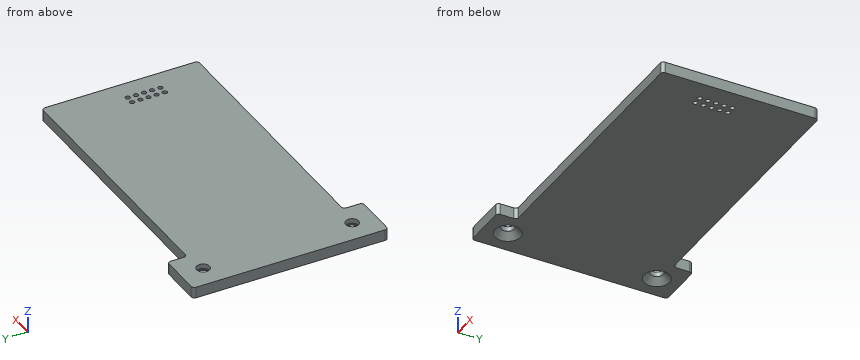
Autodesk Inventor part; units mm, degrees
ref_plane "YZ Plane" through (0, 0, 0) normal (1, 0, 0) x (0, 1, 0)
ref_plane "XZ Plane" through (0, 0, 0) normal (0, 1, 0) x (-1, 0, 0)
ref_plane "XY Plane" through (0, 0, 0) normal (0, 0, 1) x (1, 0, 0)
sketch "Boceto1" plane through (0, 0, 0) normal (0, 0, 1) x (1, 0, 0)
  line L0 (-26, 17) -> (26, 17)
  line L1 (26, 17) -> (26, -17)
  line L2 (26, -17) -> (-26, -17)
  line L3 (-26, -17) -> (-26, 17)
  line L4 (-26, 17) -> (26, -17) construction
  line L5 (26, 17) -> (-26, -17) construction
  point P0 (0, 0)
  dimension "d0" = 52
  dimension "d1" = 34
extrude "Extrusión1" add sketch "Boceto1" against normal blind 1.742
fillet "Empalme1" radius 0.5 4 edges at (26, 17, -0.871) (-26, 17, -0.871) (-26, -17, -0.871) (26, -17, -0.871)
sketch "Boceto2" plane through (0, 0, -1.742) normal (0, 0, -1) x (-1, 0, 0)
  line L0 (-25.5, 17) -> (25.5, 17)
  line L1 (25.5, -17) -> (-25.5, -17)
  line L2 (25.5, 17) -> (-25.5, 17)
  line L3 (15.5, 17) -> (-26, 17)
  line L4 (-26, 17) -> (-26, 12.2)
  line L5 (-26, 12.2) -> (15.5, 12.2)
  line L6 (15.5, 12.2) -> (15.5, 17)
  line L7 (-26, -16.5) -> (-26, 16.5)
  line L8 (-25.5, -17) -> (25.5, -17)
  line L9 (-26, 16.5) -> (-26, -16.5)
  line L10 (15.5, -17) -> (-26, -17)
  line L11 (-26, -17) -> (-26, -12.2)
  line L12 (-26, -12.2) -> (15.5, -12.2)
  line L13 (15.5, -12.2) -> (15.5, -17)
  point P0 (0, 0)
  dimension "d5" = 4.8
  dimension "d6" = 41.5
  dimension "d7" = 4.8
  dimension "d8" = 41.5
extrude "Extrusión2" cut sketch "Boceto2" against normal through all
sketch "Boceto4" plane through (0, 0, 0) normal (0, 0, 1) x (1, 0, 0)
  line L0 (-26, -16.5) -> (-26, 16.5) construction
  line L1 (-26, 17) -> (-22.8, 17)
  line L2 (-22.8, 17) -> (-22.8, -17)
  line L3 (-22.8, -17) -> (-26, -17)
  line L4 (-26, -17) -> (-26, 17)
  line L5 (-15.5, -17) -> (-25.5, -17)
  line L6 (-25.5, 17) -> (-15.5, 17)
  point P0 (0, 0)
  dimension "d17" = 3.2
extrude "Extrusión4" cut sketch "Boceto4" against normal up to surface (1.742 mm away)
sketch "Boceto7" plane through (0, 0, -1.742) normal (0, 0, -1) x (-1, 0, 0)
  line L0 (22.8, -17) -> (22.8, 17)
  line L1 (22.8, 17) -> (15.5, 17)
  line L2 (15.5, -17) -> (22.8, -17)
  point P0 (0, 0)
  point P1 (19.1, 11.638)
  point P2 (19.1, -11.638)
  dimension "d30" = 3.7
  dimension "d31" = 5.362
  dimension "d32" = 5.362
hole "Agujero2" at (-19.1, 11.638, -1.742) at (-19.1, -11.638, -1.742) direction (0, 0, 1) diameter 2 end through all countersink diameter 4 countersink angle 90
fillet "Empalme2" radius 0.5 8 edges at (-15.5, 17, -0.871) (-22.8, 17, -0.871) (-15.5, 12.2, -0.871) (26, 12.2, -0.871) (26, -12.2, -0.871) (-15.5, -12.2, -0.871) (-15.5, -17, -0.871) (-22.8, -17, -0.871)
sketch "Boceto8" plane through (0, 0, -1.742) normal (0, 0, -1) x (-1, 0, 0)
  line L0 (-26, 11.7) -> (-26, -11.7) construction
  line L1 (-25.5, -12.2) -> (15, -12.2) construction
  circle A0 centre (-22.735, 0.54) radius 0.37
  circle A1 centre (-21.465, 0.54) radius 0.37
  circle A2 centre (-22.735, -0.73) radius 0.37
  circle A3 centre (-21.465, -0.73) radius 0.37
  circle A4 centre (-22.735, -2) radius 0.37
  circle A5 centre (-21.465, -2) radius 0.37
  circle A6 centre (-22.735, -3.27) radius 0.37
  circle A7 centre (-21.465, -3.27) radius 0.37
  circle A8 centre (-22.735, -4.54) radius 0.37
  circle A9 centre (-21.465, -4.54) radius 0.37
  point P0 (0, 0)
  dimension "d49" = 3.265
  dimension "d50" = 1.27
  dimension "d51" = 1.27
  dimension "d52" = 1.27
  dimension "d53" = 1.27
  dimension "d54" = 12.74
  dimension "d55" = 0.74
  dimension "d56" = 0.74
  dimension "d57" = 0.74
  dimension "d58" = 0.74
  dimension "d59" = 0.74
  dimension "d60" = 0.74
  dimension "d61" = 0.74
  dimension "d62" = 0.74
  dimension "d63" = 1.27
  dimension "d64" = 0.74
  dimension "d65" = 0.74
extrude "Extrusión5" cut sketch "Boceto8" against normal up to surface (1.742 mm away)
sketch "Boceto9" plane through (0, 0, -1.742) normal (0, 0, -1) x (-1, 0, 0)
  line L0 (22.8, -17) -> (15.5, -17)
  line L1 (15.5, -17) -> (15.5, -15.258)
  line L2 (15.5, -15.258) -> (22.8, -15.258)
  line L3 (22.8, -15.258) -> (22.8, -17)
  line L4 (22.8, 15.258) -> (15.5, 15.258)
  line L5 (15.5, 15.258) -> (15.5, 17)
  line L6 (15.5, 17) -> (22.8, 17)
  line L7 (22.8, 17) -> (22.8, 15.258)
  point P0 (0, 0)
  point P1 (22.3, -17)
  point P2 (22.8, -16.5)
  point P3 (15.5, -16.5)
  point P4 (16, 17)
  point P5 (22.8, 16.5)
  point P6 (15.5, 16.5)
  dimension "d43" = 1.742
  dimension "d44" = 1.742
extrude "Extrusión6" cut sketch "Boceto9" against normal up to surface (1.742 mm away)
fillet "Empalme3" radius 0.5 4 edges at (-22.8, -15.258, -0.871) (-15.5, -15.258, -0.871) (-22.8, 15.258, -0.871) (-15.5, 15.258, -0.871)
properties part number "hw_DAA - PCB Peripherals" material "PCB"
The listing builds one solid part. Answer for the finished solid, in the listing's coordinates (mm). Give positions to 0.01 mm unless a question says otherwise; leave off trailing zeros. Write each loop counter-clockwise with the first axis right and the second up, starting at its lowest first coordinate (ties: lowest second). Pieces come first, ordered by that corner, then holes. Notation, with made-up numbers: (-37.5, 77) -> (4.5, 77) arc R27 ccw to (4.5, 111) -> close; hole circle Ø4 at (68, -1.5). An arc over 180 degrees is marked (long way). One line per question, with ' | ' between items. Start each with the question number.
1. Find the intervals of material crossed by probe 1 along Y at (x, z) = (-19.1, -0.6); probe 2 along Y at (x, z) = (23.5, -0.1); probe 3 along X at (y, z) = (-3, -0.5), in increasing order.
2. Section B-B (x = -6.5) is taken. Determine the outline of the cut face in (y, z).
3. Given pin 1 Ø0.5 at (y, z) = (-14, -1.5) entering from +X; pin 2 Ø1.2 at (x, y) = (-19.1, -11.638) entering from -Z; pin 3 Ø0.9 at (x, z) = (4.5, -1) entering from +Y, each flat-ended and moving along its own axis, determine where each tip first touches the part or whether it passes through.
4. Section A-A (z = -0.35) is taken. State how many separate pieces and enclosed holes the cut face has, plus the area to 3 significant figures.
Response values:
1) probe 1: -15.26 to -12.64, -10.64 to 10.64, 12.64 to 15.26 | probe 2: -12.2 to 12.2 | probe 3: -22.8 to 21.21, 21.72 to 22.48, 22.99 to 26
2) outline: (-12.2, -1.74) -> (12.2, -1.74) -> (12.2, 0) -> (-12.2, 0) -> close
3) pin 1: x = -15.5 | pin 2: through | pin 3: y = 12.2
4) separate pieces: 1 | enclosed holes: 12 | area: 1,220 mm2
